Build history of the part. All positions in model axes, mm. Round coordinates to 2 decimals unless told otherwise and drop trailing zeros. Write each loop counter-clockwise with the first axis right and the second up, starting at its lowest first coordinate (ties: lowest second). Pieces come first, ordered by that corner, then holes. Notation, with made-up numbers: M 50,25.5 L 63,25.5 A21 cw 63,46.5 Z; hole C 35,16.5 d7. An arc over 180 degrees is marked long. Write item = value, one per line.
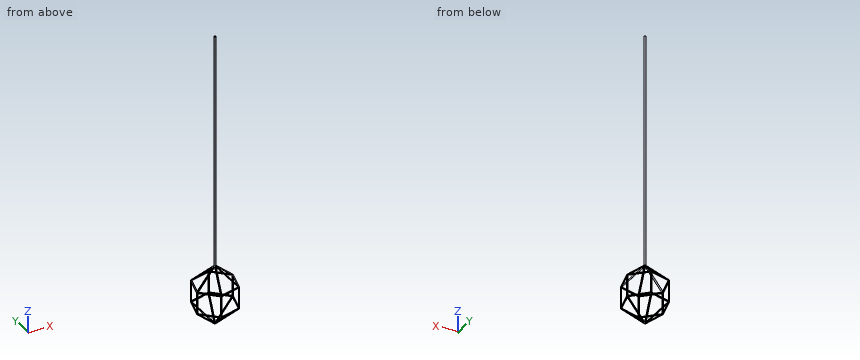
from build123d import *

# Parameters (mm, degrees)
F1_DEPTH  = 203.2
F2_SIZE   = 63.5
F3_T      = -2.54
F5_DEPTH  = 2.54
F7_DEPTH  = 2.54
F9_DEPTH  = 7.1852048969
F10_DEPTH = 2.541
F12_DEPTH = 2.54
F14_DEPTH = 2.54
F15_W     = 71.12
F15_H     = 71.12
F16_DEPTH = 157.0594794416
F17_W     = 71.12
F17_H     = 71.12
F18_DEPTH = 155.1690173594
F19_W     = 71.12
F19_H     = 71.12
F20_DEPTH = 170.067634702
F22_DEPTH = 2.54
F24_DEPTH = 2.54
F26_DEPTH = 2.54
F28_DEPTH = 2.54
F30_DEPTH = 2.54
F32_DEPTH = 2.54
F33_R     = 2.54
F34_DEPTH = 800


# Not quite as in the source:
# - a feature names something its author has since deleted; it is built from what else it names


with BuildPart() as f1:
    # F0 (on Top) → F1 (new body)
    with BuildSketch(Plane.XY):
        Polygon((73.3134762531, 20.774364002), (18.6656111534, 73.8785148759), (-54.6478650997, 53.104150874), (-73.3134762531, -20.774364002), (-18.6656111534, -73.8785148759), (54.6478650997, -53.104150874), align=None)
    extrude(amount=F1_DEPTH)

    # F2
    f2_edges = [f1.edges().sort_by_distance(p)[0] for p in [
        (45.989544, 47.326439, 203.2),
        (-17.991127, 63.491333, 203.2),
        (-63.980671, 16.164893, 203.2),
        (-45.989544, -47.326439, 203.2),
        (17.991127, -63.491333, 203.2),
        (63.980671, -16.164893, 203.2),
        (45.989544, 47.326439, 0),
        (-17.991127, 63.491333, 0),
        (-63.980671, 16.164893, 0),
        (-45.989544, -47.326439, 0),
        (17.991127, -63.491333, 0),
        (63.980671, -16.164893, 0),
    ]]
    chamfer(f2_edges, length=F2_SIZE)

    # F3
    f3_openings = [f1.faces().sort_by_distance(p)[0] for p in [
        (-42.712352, 10.791394, 161.636633),
    ]]
    offset(amount=F3_T, openings=f3_openings)

    # F4 (on face) → F5 (cut, through all)
    with BuildSketch(Plane(origin=(-71.6735768194, -73.7570960609, 102.8455678842), x_dir=(0.8701504485, -0.287188723, 0.4004507889), z_dir=(-0.4927861574, -0.5071112335, 0.7071067812))):
        Polygon((2.6696402664, 64.4858378393), (59.2408259088, 25.6139572621), (78.5633694658, 114.3351670347), align=None)
    extrude(amount=-F5_DEPTH, mode=Mode.SUBTRACT)

    # F6 (on face) → F7 (cut, through all)
    with BuildSketch(Plane(origin=(28.0387304884, -98.9496863361, 102.8455678842), x_dir=(0.9812423716, 0.1336581106, -0.1389205444), z_dir=(0.192778132, -0.6803209476, 0.7071067812))):
        Polygon((-44.3893807317, 46.8522479636), (22.9119959884, 60.3373077027), (-27.2544501276, 136.0217938087), align=None)
    extrude(amount=-F7_DEPTH, mode=Mode.SUBTRACT)

    # F8 (on face) → F9 (cut, through all)
    with BuildSketch(Plane(origin=(99.7123073078, -25.1925902753, 102.8455678842), x_dir=(0.7280120913, 0.1631104703, -0.6658778937), z_dir=(0.6855642894, -0.1732097142, 0.7071067812))):
        Polygon((-133.1636625665, 49.1073482105), (-134.131528973, 46.3985518281), (-61.9006782251, -18.3416021227), (-36.2615283041, 53.4154462512), align=None)
        Polygon((-63.0205602981, -13.9269250267), (-130.6368034196, 46.6771789529), (-39.925449456, 50.7100458165), align=None, mode=Mode.SUBTRACT)
    extrude(amount=-F9_DEPTH, mode=Mode.SUBTRACT)

    # F8 (on face) + F2_face2 (on face) → F10 (cut, through all)
    with BuildSketch(Plane(origin=(99.7123073078, -25.1925902753, 102.8455678842), x_dir=(0.7280120913, 0.1631104703, -0.6658778937), z_dir=(0.6855642894, -0.1732097142, 0.7071067812))):
        Polygon((-133.1636625665, 49.1073482105), (-134.131528973, 46.3985518281), (-61.9006782251, -18.3416021227), (-36.2615283041, 53.4154462512), align=None)
        Polygon((-63.0205602981, -13.9269250267), (-130.6368034196, 46.6771789529), (-39.925449456, 50.7100458165), align=None, mode=Mode.SUBTRACT)
    with BuildSketch(Plane(origin=(42.71235225, -10.7913939511, 161.636632955), x_dir=(0.2449555269, 0.969534316, 0), z_dir=(0.6855642894, -0.1732097142, 0.7071067812))):
        Polygon((-34.3195357799, -28.4830838377), (34.3195357799, -28.4830838377), (0, 55.5822670322), align=None)
    extrude(amount=-F10_DEPTH, mode=Mode.SUBTRACT)

    # F11 (on face) → F12 (cut, through all)
    with BuildSketch(Plane(origin=(71.6735768194, 73.7570960609, 102.8455678842), x_dir=(0.8701504485, -0.287188723, -0.4004507889), z_dir=(0.4927861574, 0.5071112335, 0.7071067812))):
        Polygon((-59.2408259088, -25.6139572621), (-78.5633694658, -114.3351670347), (-2.6696402664, -64.4858378393), align=None)
    extrude(amount=-F12_DEPTH, mode=Mode.SUBTRACT)

    # F13 (on face) → F14 (cut, through all)
    with BuildSketch(Plane(origin=(-28.0387304884, 98.9496863361, 102.8455678842), x_dir=(0.9812423716, 0.1336581106, 0.1389205444), z_dir=(-0.192778132, 0.6803209476, 0.7071067812))):
        Polygon((44.3893807317, -46.8522479636), (-22.9119959884, -60.3373077027), (27.2544501276, -136.0217938087), align=None)
    extrude(amount=-F14_DEPTH, mode=Mode.SUBTRACT)

    # F15 (on face) → F16 (cut, through all)
    with BuildSketch(Plane(origin=(17.9911269732, -63.4913328749, 0), x_dir=(0.9621191109, 0.2726294488, 0), z_dir=(0.2726294488, -0.9621191109, 0))):
        with Locations((0, 101.6)):
            Rectangle(F15_W, F15_H)
    extrude(amount=-F16_DEPTH, mode=Mode.SUBTRACT)

    # F17 (on face) → F18 (cut, through all)
    with BuildSketch(Plane(origin=(63.9806706764, -16.164893436, 0), x_dir=(0.2449555269, 0.969534316, 0), z_dir=(0.969534316, -0.2449555269, 0))):
        with Locations((0, 101.6)):
            Rectangle(F17_W, F17_H)
    extrude(amount=-F18_DEPTH, mode=Mode.SUBTRACT)

    # F19 (on face) → F20 (cut, through all)
    with BuildSketch(Plane(origin=(45.9895437032, 47.3264394389, 0), x_dir=(-0.717163584, 0.6969048671, 0), z_dir=(0.6969048671, 0.717163584, 0))):
        with Locations((0, 101.6)):
            Rectangle(F19_W, F19_H)
    extrude(amount=-F20_DEPTH, mode=Mode.SUBTRACT)

    # F21 (on face) → F22 (cut, through all)
    with BuildSketch(Plane(origin=(1.2076208066, -0.3051087374, -1.2455678842), x_dir=(0.7280120913, 0.1631104703, 0.6658778937), z_dir=(0.6855642894, -0.1732097142, -0.7071067812))):
        Polygon((95.3809385521, -2.3644010884), (72.2858277101, 62.2725697547), (4.6695845886, 1.6684657751), align=None)
    extrude(amount=-F22_DEPTH, mode=Mode.SUBTRACT)

    # F23 (on face) → F24 (cut, through all)
    with BuildSketch(Plane(origin=(0.8680423208, 0.8932759279, -1.2455678842), x_dir=(0.8701504485, -0.287188723, 0.4004507889), z_dir=(0.4927861574, 0.5071112335, -0.7071067812))):
        Polygon((22.13077439, -92.8080958564), (78.7019600324, -53.9362152793), (2.808230833, -4.0868860838), align=None)
    extrude(amount=-F24_DEPTH, mode=Mode.SUBTRACT)

    # F25 (on face) → F26 (cut, through all)
    with BuildSketch(Plane(origin=(-0.3395784858, 1.1983846653, -1.2455678842), x_dir=(0.9812423716, 0.1336581106, -0.1389205444), z_dir=(-0.192778132, 0.6803209476, -0.7071067812))):
        Polygon((16.1607261154, -94.0316157631), (-0.9742044888, -4.862069918), (-51.1406506047, -80.546556024), align=None)
    extrude(amount=-F26_DEPTH, mode=Mode.SUBTRACT)

    # F27 (on face) → F28 (cut, through all)
    with BuildSketch(Plane(origin=(-1.2076208066, 0.3051087374, -1.2455678842), x_dir=(0.7280120913, 0.1631104703, -0.6658778937), z_dir=(-0.6855642894, 0.1732097142, -0.7071067812))):
        Polygon((-72.2858277101, -62.2725697547), (-4.6695845886, -1.6684657751), (-95.3809385521, 2.3644010884), align=None)
    extrude(amount=-F28_DEPTH, mode=Mode.SUBTRACT)

    # F29 (on face) → F30 (cut, through all)
    with BuildSketch(Plane(origin=(-0.8680423208, -0.8932759279, -1.2455678842), x_dir=(0.8701504485, -0.287188723, -0.4004507889), z_dir=(-0.4927861574, -0.5071112335, -0.7071067812))):
        Polygon((-78.7019600324, 53.9362152793), (-2.808230833, 4.0868860838), (-22.13077439, 92.8080958564), align=None)
    extrude(amount=-F30_DEPTH, mode=Mode.SUBTRACT)

    # F31 (on face) → F32 (cut, through all)
    with BuildSketch(Plane(origin=(0.3395784858, -1.1983846653, -1.2455678842), x_dir=(0.9812423716, 0.1336581106, 0.1389205444), z_dir=(0.192778132, -0.6803209476, -0.7071067812))):
        Polygon((-16.1607261154, 94.0316157631), (0.9742044888, 4.862069918), (51.1406506047, 80.546556024), align=None)
    extrude(amount=-F32_DEPTH, mode=Mode.SUBTRACT)

    # F33 (on face) → F34 (join)
    with BuildSketch(Plane.XY.offset(203.2)):
        Circle(F33_R)
    extrude(amount=F34_DEPTH)


solid = f1.part
1. Flat gauge pins, fed straight in: pin 1 (17.5 mm diameter, centred on x = 2, y = -57, fed in from -Z); pin 2 (6.5 mm diameter, centred on x = -26, y = 60.5, fed in from +Z); pin 3 (3 mm diameter, centred on x = -52, y = 44.5, fed in from -Z). Where does each tip first touch, or does it go through?
Responses:
pin_1 = 61.76
pin_2 = 141.5
pin_3 = 63.08
2. Band-saw the part on A-A (z = 163). List the corners of the cut face in (x, y).
Responses:
outline = M -47.43,-13.44 L -45.46,-15.35 L -42.21,-13.5 L -46.41,-9.42 Z; M -36.37,30.33 L -30.74,31.93 L -32.71,35.1 L -35.35,34.35 Z; M -14.04,-45.88 L -12.08,-47.79 L -9.44,-47.05 L -9.42,-43.31 L -11.06,-43.77 L -12.28,-42.58 Z; M 9.42,43.31 L 11.06,43.77 L 12.28,42.58 L 14.04,45.88 L 12.08,47.79 L 9.44,47.05 Z; M 30.74,-31.93 L 32.71,-35.1 L 35.35,-34.35 L 31.05,-31.84 Z; M 42.21,13.5 L 42.45,13.27 L 47.43,13.44 L 45.46,15.35 Z
3. Probe probe 1 along Z at (x, y) = (-51, -38.5); probe 2 along Z at (x, y) = (-60.5, -14). List the from-to ranges inside material, lowest first.
Responses:
probe_1 = 62.75 to 64.25, 138.95 to 140.45
probe_2 = 149.9 to 150.46
4. Band-saw the part on C-C (z = 896). List the corners of the cut face in (x, y), plus the area to 3 significant figures.
Responses:
outline = C 0,0 d5.08
area = 20.3 mm²
5. Band-saw the part on B-B (x = -30.5). Count the separate pieces of the cut face and the enclosed holes in it, plus the area to 3 significant figures.
Responses:
separate_pieces = 8
enclosed_holes = 0
area = 116 mm²
